Verification items for the finished model (mm, model axes). A direction names the side the tool comes from. Give positions to 0.01 mm unless a question says otherwise; leave off trailing zeros. Loops run counter-clockwise (first coordinate to the right, second up) from the corner with the lowest first, then second, coordinate; pieces in that order, holes last. Notation, with made-up numbers: (72, 1) -> (97, 1) arc R13 ccw to (97, 8) -> close; hole circle Ø10 at (21, -5). An arc over 180 degrees is marked (long way). Answer in a Markdown table with one row per item. Add a question column.
Q1. Material ranges on probe 1 along Y at (x, z) = (0, 3); probe 2 along X at (y, z) = (12, 5.25); probe 3 along Y at (x, z) = (3.5, 6.5), recorded low to high.
Q2. Release check for a two-part mould opening along Y. For faces 1 (the face through (0.2, -35, 3.9)), 2 (the face through (-0.651, -21.525, 4.056)), 3 (the face through (10, 76, 4)) record: pulls with the +Y half, pulls with the -Y half, needs draft (parallel to the pull), parting line crosses it, or undercut.
Q3. Section check A-A on x = 0. Enter the section's corners in (y, z), and give its area (3 significant figures).
Q4. Section check B-B on y = 81.5. Enter the section's corners in (x, z).
Q5. Gauge pin test, flat ends, axial feed: P1, Ø1, axis at x = -2.5, z = 6, coming from the -Y side; P2, Ø2, axis at x = -7, z = 6.5, coming from the +Y side; P3, Ø6, axis at x = -8, y = 85, coming from the -Z side. Record the tip position at first contact, or that the pin passes through.
Q6. Set-up check for faces 4 (the face through (-4.3, 76.5, 0)), 5 (the face through (0.088, 0.997, 3.944)): record each of +Z, -Z, +X, -X, +Y, -Y from which the full face is reachable in a straight line by a thin tool's end or side.
Q7. Section check C-C on z = 1.75. Enter the section's corners in (x, y), and give its area (3 significant figures).
```python
from build123d import *

# Parameters (mm, degrees)
BOSS_EXTRUDE1_DEPTH = 8
SKETCH3_R           = 5
CUT_EXTRUDE1_DEPTH  = 8


with BuildPart() as part:
    # Sketch2 → Boss-Extrude1 (new body)
    with BuildSketch(Plane.XY):
        with BuildLine():
            Line((10, 174.996075103), (10, -25.003924897))
            ThreePointArc((10, -25.003924897), (0, -35.003924897), (-10, -25.003924897))
            Line((-10, -25.003924897), (-10, 174.996075103))
            ThreePointArc((-10, 174.996075103), (0, 184.996075103), (10, 174.996075103))
        make_face()
        with BuildLine():
            Line((4, 174.996075103), (4, 4.996075103))
            ThreePointArc((4, 4.996075103), (0, 0.996075103), (-4, 4.996075103))
            Line((-4, 4.996075103), (-4, 174.996075103))
            ThreePointArc((-4, 174.996075103), (0, 178.996075103), (4, 174.996075103))
        make_face(mode=Mode.SUBTRACT)
    extrude(amount=BOSS_EXTRUDE1_DEPTH)

    # Sketch3 → Cut-Extrude1 (cut)
    with BuildSketch(Plane.XY.offset(8)):
        with Locations((0, -26.482483783)):
            Circle(SKETCH3_R)
    extrude(amount=-CUT_EXTRUDE1_DEPTH, mode=Mode.SUBTRACT)


solid = part.part
```
Taken from the geometry:
| question | item | result |
|---|---|---|
| 1 | probe 1 | y = -35 to -31.48, -21.48 to 1, 179 to 185 |
| 1 | probe 2 | x = -10 to -4, 4 to 10 |
| 1 | probe 3 | y = -34.37 to -30.05, -22.91 to 3.06, 176.93 to 184.36 |
| 2 | face 1 | pulls with the -Y half |
| 2 | face 2 | undercut |
| 2 | face 3 | needs draft |
| 3 | outline | (-35, 0) -> (-31.48, 0) -> (-31.48, 8) -> (-35, 8) -> close; (-21.48, 0) -> (1, 0) -> (1, 8) -> (-21.48, 8) -> close; (179, 0) -> (185, 0) -> (185, 8) -> (179, 8) -> close |
| 3 | area | 256 mm² |
| 4 | outline | (-10, 0) -> (-4, 0) -> (-4, 8) -> (-10, 8) -> close; (4, 0) -> (10, 0) -> (10, 8) -> (4, 8) -> close |
| 5 | P1 | stops at y = -34.8 |
| 5 | P2 | stops at y = 183 |
| 5 | P3 | stops at z = 0 |
| 6 | face 4 | -Z, +X, -X, +Y, -Y |
| 6 | face 5 | +Z, -Z |
| 7 | outline | (-10, -25) arc R10 ccw to (10, -25) -> (10, 175) arc R10 ccw to (-10, 175) -> close; hole circle Ø10 at (0, -26.48); hole (-4, 5) arc R4 ccw to (4, 5) -> (4, 175) arc R4 ccw to (-4, 175) -> close |
| 7 | area | 2,830 mm² |
